Work out the finished part from the listing and answer in its coordinate system (mm). A direction names the side the tool comes from. Round coordinates to 2 decimals unless told otherwise and drop trailing zeros. Loops run counter-clockwise (first coordinate to the right, second up) from the corner with the lowest first, then second, coordinate; pieces in that order, holes last.
```python
from build123d import *

# Parameters (mm, degrees)
ESBO_O1_R                = 1.75
RESSALTO_EXTRUS_O1_DEPTH = 5


with BuildPart() as part:
    # Esboço1 → Ressalto-extrusão1 (new body)
    with BuildSketch(Plane.XY):
        with BuildLine():
            Line((67.25, 10), (67.25, -10))
            ThreePointArc((67.25, -10), (65.553481285, -13.864617802), (61.560373044, -15.231560775))
            Line((61.560373044, -15.231560775), (-57.439626956, -5.231560775))
            ThreePointArc((-57.439626956, -5.231560775), (-62.25, 0), (-57.439626956, 5.231560775))
            Line((-57.439626956, 5.231560775), (61.560373044, 15.231560775))
            ThreePointArc((61.560373044, 15.231560775), (65.553481285, 13.864617802), (67.25, 10))
        make_face()
        with Locations((62, -10)):
            Circle(ESBO_O1_R, mode=Mode.SUBTRACT)
        with Locations(Location((62, 10, 0), (0, 0, 180))):
            Circle(ESBO_O1_R, mode=Mode.SUBTRACT)
        with BuildLine():
            Line((47, -1.75), (37, -1.75))
            ThreePointArc((37, -1.75), (35.25, 0), (37, 1.75))
            Line((37, 1.75), (47, 1.75))
            ThreePointArc((47, 1.75), (48.75, 0), (47, -1.75))
        make_face(mode=Mode.SUBTRACT)
        with BuildLine():
            Line((-47, -1.75), (-57, -1.75))
            ThreePointArc((-57, -1.75), (-58.75, 0), (-57, 1.75))
            Line((-57, 1.75), (-47, 1.75))
            ThreePointArc((-47, 1.75), (-45.25, 0), (-47, -1.75))
        make_face(mode=Mode.SUBTRACT)
    extrude(amount=RESSALTO_EXTRUS_O1_DEPTH)


solid = part.part
```
1. Find section C-C (x = 20). Write down the section's boundary in (y, z).
Answer key:
outline: (-11.74, 0) - (11.74, 0) - (11.74, 5) - (-11.74, 5) - close
2. Consider probe 1 along Y at (x, z) = (62, 2); probe 2 along X at (y, z) = (1.5, 3.7); probe 3 along Y at (x, z) = (-56, 2.7). Determine where each line is inside the solid, lowest interval first.
Answer key:
probe 1: y = -15.25 to -11.75, -8.25 to 8.25, 11.75 to 15.25
probe 2: x = -62.03 to -57.9, -46.1 to 36.1, 47.9 to 67.25
probe 3: y = -5.35 to -1.75, 1.75 to 5.35
3. Find section D-D (y = 13). Write down the section's boundary in (x, z).
Answer key:
outline: (35, 0) - (66.31, 0) - (66.31, 5) - (35, 5) - close
4. Given pin 1 (2.5 mm diameter, centred on x = 40.5, z = 3, fed in from -Y); pin 2 (3 mm diameter, centred on x = -37.5, z = 2, fed in from -Y); pin 3 (3 mm diameter, centred on x = -5.5, z = 1, fed in from -Y), each flat-ended and moving along its own axis, determine where each tip first touches the part or whether it passes through.
Answer key:
pin 1: stops at y = -13.57
pin 2: stops at y = -7.03
pin 3: stops at y = -9.72
5. Find section B-B (z = 2.3). Write down the section's boundary in (x, y).
Answer key:
outline: (-57.44, -5.23) - (61.56, -15.23) arc R5.25 ccw to (67.25, -10) - (67.25, 10) arc R5.25 ccw to (61.56, 15.23) - (-57.44, 5.23) arc R5.25 ccw to start; hole (-57, -1.75) - (-47, -1.75) arc R1.75 ccw to (-47, 1.75) - (-57, 1.75) arc R1.75 ccw to start; hole (37, -1.75) - (47, -1.75) arc R1.75 ccw to (47, 1.75) - (37, 1.75) arc R1.75 ccw to start; hole circle Ø3.5 at (62, -10); hole circle Ø3.5 at (62, 10)
6. Find section A-A (y = 0). Write down the section's boundary in (x, z), then the cut area to 4 significant figures.
Answer key:
outline: (-62.25, 0) - (-58.75, 0) - (-58.75, 5) - (-62.25, 5) - close; (-45.25, 0) - (35.25, 0) - (35.25, 5) - (-45.25, 5) - close; (48.75, 0) - (67.25, 0) - (67.25, 5) - (48.75, 5) - close
area: 512.5 mm2
7. Determine the mould class of faces 1 (the face through (18, 0, 5)), 2 (the face through (-62.25, -0.11, 2.46)), 3 (the face through (42, 1.75, 2)) for opening direction X: +X half, -X half, draft (parallel to the pull), parting line (faces both ways), or undercut.
Answer key:
face 1: draft
face 2: -X half
face 3: undercut
8. Which of the six approach directions +Z, -Z, +X, -X, +Y, -Y give full straight-line access (tool end or side, diameter ignored) to faces 4 (the face through (35.25, -0.04, 2.46)), 5 (the face through (1.23, 10.16, 2.46))?
Answer key:
face 4: +Z, -Z
face 5: +Z, -Z, -X, +Y
